Could you check a few things on this model? Use its own coordinates, in mm. Face numbers are marked on the shaded views. A direction names the side the tool comes from. Round coordinates to 2 decimals unless told otherwise and drop trailing zeros. Loops run counter-clockwise (first coordinate to the right, second up) from the corner with the lowest first, then second, coordinate; pieces in that order, holes last. Notation, with made-up numbers: (70.25, 64.25) -> (84.25, 64.25) arc R32 cw to (84.25, 90.25) -> close; hole circle Ø11 at (4.5, 51.25). An arc over 180 degrees is marked (long way). Write each question's results on one line, items separated by ' | '.
from build123d import *

# Parameters (mm, degrees)
SKETCH1_R           = 13.97
BOSS_EXTRUDE1_DEPTH = 19.05
SKETCH2_R           = 4.6355
BOSS_EXTRUDE2_DEPTH = 1.4605
SKETCH3_R           = 2.4765
BOSS_EXTRUDE3_DEPTH = 7.8232
CUT_EXTRUDE1_DEPTH  = 6.2611
SKETCH6_R           = 13.97
SKETCH6_R_2         = 2.0828
BOSS_EXTRUDE4_DEPTH = 0.8382
BOSS_EXTRUDE5_DEPTH = 16.0528
BOSS_EXTRUDE6_DEPTH = 13.208
SKETCH9_R           = 2.4765
CUT_EXTRUDE2_DEPTH  = 10.6934


with BuildPart() as part:
    # Sketch1 → Boss-Extrude1 (new body)
    with BuildSketch(Plane(origin=(0, 0, 0), x_dir=(1, 0, 0), z_dir=(0, 1, 0))):
        Circle(SKETCH1_R)
    extrude(amount=BOSS_EXTRUDE1_DEPTH)

    # Sketch2 → Boss-Extrude2 (add)
    with BuildSketch(Plane(origin=(0, 19.05, 0), x_dir=(1, 0, 0), z_dir=(0, 1, 0))):
        with Locations((0, 7.6581)):
            Circle(SKETCH2_R)
    extrude(amount=BOSS_EXTRUDE2_DEPTH)

    # Sketch3 → Boss-Extrude3 (add)
    with BuildSketch(Plane(origin=(0, 20.5105, 0), x_dir=(1, 0, 0), z_dir=(0, 1, 0))):
        with Locations((0, 7.6581)):
            Circle(SKETCH3_R)
    extrude(amount=BOSS_EXTRUDE3_DEPTH)

    # Sketch5 → Cut-Extrude1 (cut)
    with BuildSketch(Plane(origin=(0, 28.3337, 0), x_dir=(1, 0, 0), z_dir=(0, 1, 0))):
        with BuildLine():
            ThreePointArc((1.999998, 9.1186), (0, 10.1346), (-1.999998, 9.1186))
            Line((-1.999998, 9.1186), (1.999998, 9.1186))
        make_face()
        with BuildLine():
            Line((1.999998, 6.1976), (-1.999998, 6.1976))
            ThreePointArc((-1.999998, 6.1976), (0, 5.1816), (1.999998, 6.1976))
        make_face()
    extrude(amount=-CUT_EXTRUDE1_DEPTH, mode=Mode.SUBTRACT)

    # Sketch6 → Boss-Extrude4 (add)
    with BuildSketch(Plane(origin=(0, 19.05, 0), x_dir=(1, 0, 0), z_dir=(0, 1, 0))):
        Circle(SKETCH6_R)
        with BuildLine():
            Line((-17.4244, 3.4671), (-13.532927163, 3.4671))
            ThreePointArc((-13.532927163, 3.4671), (-13.97, 0), (-13.532927163, -3.4671))
            Line((-13.532927163, -3.4671), (-17.4244, -3.4671))
            ThreePointArc((-17.4244, -3.4671), (-20.8915, 0), (-17.4244, 3.4671))
        make_face()
        with Locations((-17.4244, 0)):
            Circle(SKETCH6_R_2, mode=Mode.SUBTRACT)
        with BuildLine():
            Line((17.4244, 3.4671), (13.532927163, 3.4671))
            ThreePointArc((13.532927163, 3.4671), (13.97, 0), (13.532927163, -3.4671))
            Line((13.532927163, -3.4671), (17.4244, -3.4671))
            ThreePointArc((17.4244, -3.4671), (20.8915, 0), (17.4244, 3.4671))
        make_face()
        with Locations((17.4244, 0)):
            Circle(SKETCH6_R_2, mode=Mode.SUBTRACT)
    extrude(amount=-BOSS_EXTRUDE4_DEPTH)

    # Sketch7 → Boss-Extrude5 (add)
    with BuildSketch(Plane(origin=(0, 19.05, 0), x_dir=(1, 0, 0), z_dir=(0, 1, 0))):
        with BuildLine():
            Line((7.3152, -17.018), (-7.3152, -17.018))
            Line((-7.3152, -17.018), (-7.3152, -11.901627996))
            ThreePointArc((-7.3152, -11.901627996), (0, -13.97), (7.3152, -11.901627996))
            Line((7.3152, -11.901627996), (7.3152, -17.018))
        make_face()
    extrude(amount=-BOSS_EXTRUDE5_DEPTH)

    # Sketch8 → Boss-Extrude6 (add)
    with BuildSketch(Plane(origin=(0, 15.24, 0), x_dir=(1, 0, 0), z_dir=(0, 1, 0))):
        with BuildLine():
            Line((-9.0551, -10.637953938), (-9.0551, -12.258171315))
            ThreePointArc((-9.0551, -12.258171315), (0, -15.24), (9.0551, -12.258171315))
            Line((9.0551, -12.258171315), (9.0551, -10.637953938))
            ThreePointArc((9.0551, -10.637953938), (0, -13.97), (-9.0551, -10.637953938))
        make_face()
    extrude(amount=-BOSS_EXTRUDE6_DEPTH)

    # Sketch9 → Cut-Extrude2 (cut)
    with BuildSketch(Plane(origin=(0, 28.3337, 0), x_dir=(1, 0, 0), z_dir=(0, 1, 0))):
        with Locations((0, 7.6581)):
            Circle(SKETCH9_R)
    extrude(amount=-CUT_EXTRUDE2_DEPTH, mode=Mode.SUBTRACT)


solid = part.part
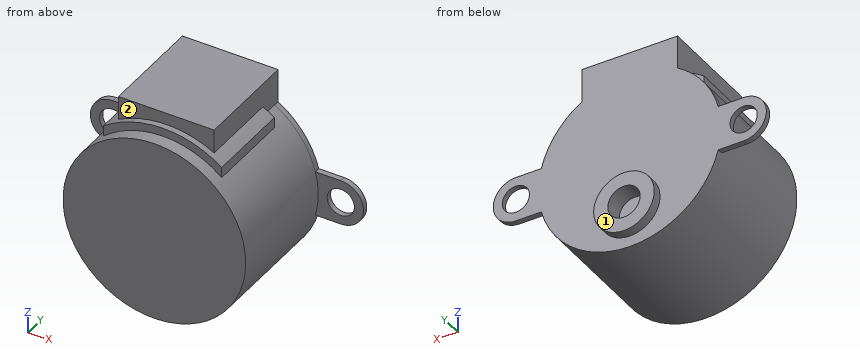
1) I want a section at D-D, the plane x = 18. Write out the boundary of the cut face in (y, z).
Model answer:
outline: (18.21, -3.42) -> (19.05, -3.42) -> (19.05, -2) -> (18.21, -2) -> close; (18.21, 2) -> (19.05, 2) -> (19.05, 3.42) -> (18.21, 3.42) -> close
2) I want a section at A-A, the plane z = 0. Write out the boundary of the cut face in (x, y).
Model answer:
outline: (-20.89, 18.21) -> (-19.51, 18.21) -> (-19.51, 19.05) -> (-20.89, 19.05) -> close; (-15.34, 18.21) -> (-13.97, 18.21) -> (-13.97, 0) -> (13.97, 0) -> (13.97, 18.21) -> (15.34, 18.21) -> (15.34, 19.05) -> (-15.34, 19.05) -> close; (19.51, 18.21) -> (20.89, 18.21) -> (20.89, 19.05) -> (19.51, 19.05) -> close
3) I'm going to push flat-ended pins straight in: pin 1 (1.5 mm diameter, centred on y = 13, z = -2.5, fed in from +X); pin 2 (8 mm diameter, centred on y = 2.5, z = 2, fed in from -X); pin 3 (1.5 mm diameter, centred on x = 0.5, z = -9, fed in from +Y); pin 4 (4 mm diameter, centred on x = -2, z = 8, fed in from -Y). Where does each tip first touch, or does it pass through?
Model answer:
pin 1: stops at x = 13.86 | pin 2: stops at x = -13.97 | pin 3: stops at y = 17.64 | pin 4: stops at y = 0
4) For the marked faces 1 and 2, which set-ups out of +Z, -Z, +X, -X, +Y, -Y let a thin tool reach every point of the face, with its end or its side?
Model answer:
face 1: +Z, -Z, +X, -X, +Y | face 2: +Z, -Y
5) I need wall thicknesses on line 1 (X direction, y = 18.7, z = 0); line 2 (Z direction, x = 0, y = 19.15); line 3 (Z direction, x = -0.5, y = 17.5). Which ranges of each line are inside material? Lowest first, please.
Model answer:
line 1: x = -20.89 to -19.51, -15.34 to 15.34, 19.51 to 20.89 | line 2: z = -12.29 to -10.13, -5.18 to -3.02 | line 3: z = -13.96 to 17.02
6) I want a section at C-C, the plane x = 0. Write out the boundary of the cut face in (y, z), plus the area to 3 significant figures.
Model answer:
outline: (0, -13.97) -> (19.05, -13.97) -> (19.05, -12.29) -> (20.51, -12.29) -> (20.51, -10.13) -> (17.64, -10.13) -> (17.64, -5.18) -> (20.51, -5.18) -> (20.51, -3.02) -> (19.05, -3.02) -> (19.05, 17.02) -> (3, 17.02) -> (3, 15.24) -> (2.03, 15.24) -> (2.03, 13.97) -> (0, 13.97) -> close | area: 582 mm2
7) I want a section at B-B, the plane y = 6.5. Write out the boundary of the cut face in (x, z), plus the area to 3 significant figures.
Model answer:
outline: (-9.06, 10.64) arc R13.97 ccw (long way) to (9.06, 10.64) -> (9.06, 12.26) arc R15.24 ccw to (7.32, 13.37) -> (7.32, 17.02) -> (-7.32, 17.02) -> (-7.32, 13.37) arc R15.24 ccw to (-9.06, 12.26) -> close | area: 673 mm2
